Source: three-view drawing plus pictorial views. Frame: mm from the lowest corner of the part. A direction names the side the tool comes from. Give positions to 0.01 mm unless a question says otherwise; leave off trailing zeros. Loops run counter-clockwise (first coordinate to the right, second up) from the corner with the lowest first, then second, coordinate; pieces in that order, holes last. Notation, with made-up numbers: (63.25, 25) -> (108.25, 25) arc R24 ccw to (108.25, 54) -> close; hole circle Ø11 at (66, 70). An arc over 180 degrees is marked (long way). Put each result on its own line as item: value.
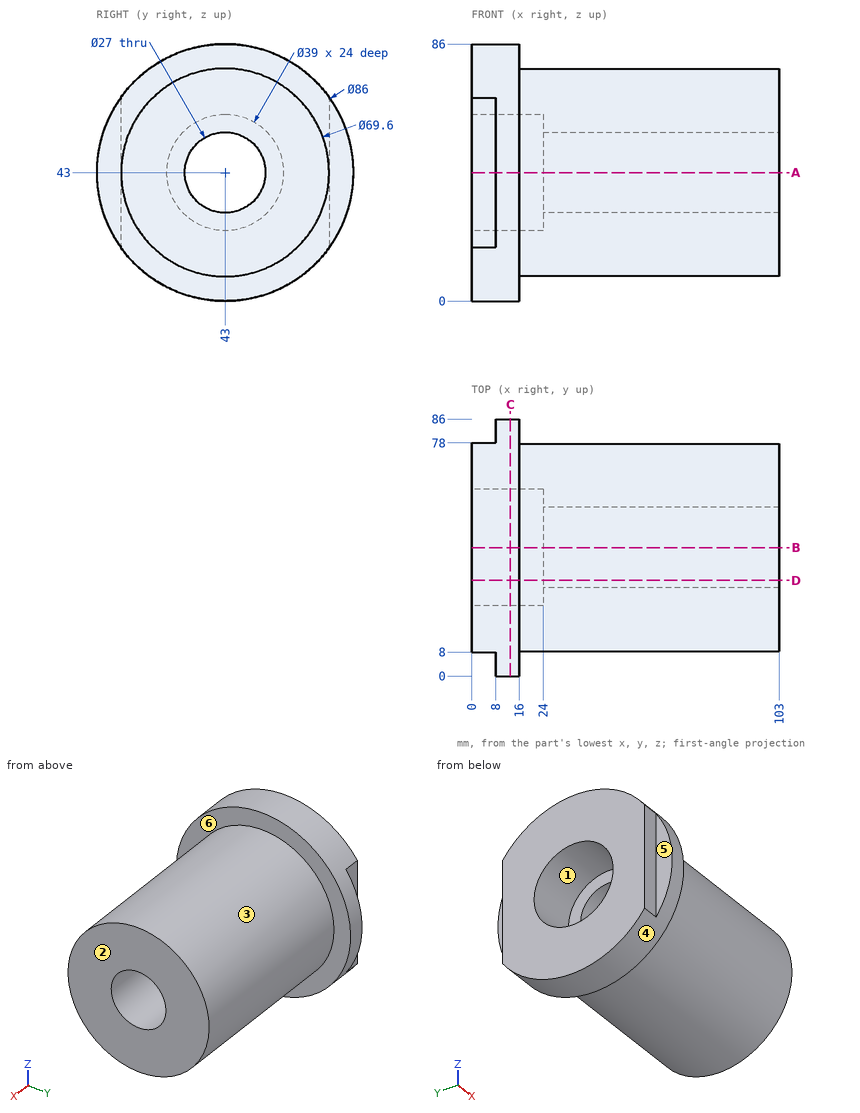
(1) Section A-A on z = 43. Return loops of the section in (x, y), then the cut area to 3 significant figures.
Calculated:
outline: (0, 8) -> (8, 8) -> (8, 0) -> (16, 0) -> (16, 8.2) -> (103, 8.2) -> (103, 29.5) -> (24, 29.5) -> (24, 23.5) -> (0, 23.5) -> close; (0, 62.5) -> (24, 62.5) -> (24, 56.5) -> (103, 56.5) -> (103, 77.8) -> (16, 77.8) -> (16, 86) -> (8, 86) -> (8, 78) -> (0, 78) -> close
area: 4,230 mm²
(2) Reachability of the marked faces 4, 5 and 6 from +Z, -Z, +X, -X, +Y, -Y: full face, straight path, thin tool, end or side. Return the list, or none.
Calculated:
face 4: +X, -X
face 5: +Z, -Z, -X, -Y
face 6: +X
(3) Draft query along Y for the marked faces 1, 2 and 3. Return one class per face: released by +Y, released by -Y, zero draft, split by the parting line, or undercut.
Calculated:
face 1: undercut
face 2: zero draft
face 3: split by the parting line
(4) First-contact query: P1, Ø6, axis at x = 50, z = 18.5, coming from the +Y side; P2, Ø21.5, axis at y = 43, z = 43, coming from the +X side; P3, Ø2.5, axis at y = 3, z = 39.5, coming from the -X side; P4, Ø4, axis at x = 4, z = 52, coming from the +Y side. Flat tips, straight axial feed; report the tip coordinate or a pass-through.
Calculated:
P1: stops at y = 70.36
P2: passes through
P3: stops at x = 8
P4: stops at y = 78
(5) Section B-B on y = 43. Return loops of the section in (x, z).
Calculated:
outline: (0, 0) -> (16, 0) -> (16, 8.2) -> (103, 8.2) -> (103, 29.5) -> (24, 29.5) -> (24, 23.5) -> (0, 23.5) -> close; (0, 62.5) -> (24, 62.5) -> (24, 56.5) -> (103, 56.5) -> (103, 77.8) -> (16, 77.8) -> (16, 86) -> (0, 86) -> close
(6) Line query: probe 1 along Y at (x, z) = (81, 43); probe 2 along Y at (x, z) = (13, 43); probe 3 along X at (y, z) = (60, 43). Output: solid intervals per line, ascending. Write a range as from..to.
Calculated:
probe 1: y = 8.2..29.5, 56.5..77.8
probe 2: y = 0..23.5, 62.5..86
probe 3: x = 24..103
(7) Section C-C on x = 13. Return loops of the section in (y, z).
Calculated:
outline: circle Ø86 at (43, 43); hole circle Ø39 at (43, 43)
(8) Section D-D on y = 32. Return loops of the section in (x, z), then the cut area to 3 significant figures.
Calculated:
outline: (0, 1.43) -> (16, 1.43) -> (16, 9.98) -> (103, 9.98) -> (103, 35.17) -> (24, 35.17) -> (24, 26.9) -> (0, 26.9) -> close; (0, 59.1) -> (24, 59.1) -> (24, 50.83) -> (103, 50.83) -> (103, 76.02) -> (16, 76.02) -> (16, 84.57) -> (0, 84.57) -> close
area: 5,070 mm²
